from build123d import *

# Parameters (mm, degrees)
BOSS_EXTRUDE1_DEPTH = 3.175
SKETCH2_W           = 11.43
SKETCH2_H           = 100.33
BOSS_EXTRUDE2_DEPTH = 1.5875


with BuildPart() as part:
    # Sketch1 → Boss-Extrude1 (new body)
    with BuildSketch(Plane.XY):
        with BuildLine():
            Line((-50.8, 171.390190343), (-50.8, 171.509809657))
            ThreePointArc((-50.8, 171.509809657), (-52.642354096, 175.957645904), (-57.090190343, 177.8))
            Line((-57.090190343, 177.8), (-190.5, 177.8))
            ThreePointArc((-190.5, 177.8), (-194.990128061, 175.940128061), (-196.85, 171.45))
            Line((-196.85, 171.45), (-196.85, 21.59))
            ThreePointArc((-196.85, 21.59), (-196.106051224, 19.793948776), (-194.31, 19.05))
            Line((-194.31, 19.05), (-193.04, 19.05))
            ThreePointArc((-193.04, 19.05), (-191.243948776, 18.306051224), (-190.5, 16.51))
            Line((-190.5, 16.51), (-190.5, 6.35))
            ThreePointArc((-190.5, 6.35), (-188.640128061, 1.859871939), (-184.15, 0))
            Line((-184.15, 0), (184.15, 0))
            ThreePointArc((184.15, 0), (188.640128061, 1.859871939), (190.5, 6.35))
            Line((190.5, 6.35), (190.5, 16.51))
            ThreePointArc((190.5, 16.51), (191.243948776, 18.306051224), (193.04, 19.05))
            Line((193.04, 19.05), (194.31, 19.05))
            ThreePointArc((194.31, 19.05), (196.106051224, 19.793948776), (196.85, 21.59))
            Line((196.85, 21.59), (196.85, 171.45))
            ThreePointArc((196.85, 171.45), (194.990128061, 175.940128061), (190.5, 177.8))
            Line((190.5, 177.8), (57.090190343, 177.8))
            ThreePointArc((57.090190343, 177.8), (52.642354096, 175.957645904), (50.8, 171.509809657))
            Line((50.8, 171.509809657), (50.8, 171.390190343))
            ThreePointArc((50.8, 171.390190343), (48.957645904, 166.942354096), (44.509809657, 165.1))
            Line((44.509809657, 165.1), (-44.509809657, 165.1))
            ThreePointArc((-44.509809657, 165.1), (-48.957645904, 166.942354096), (-50.8, 171.390190343))
        make_face()
    extrude(amount=BOSS_EXTRUDE1_DEPTH)

    # Sketch2 → Boss-Extrude2 (add)
    with BuildSketch(Plane(origin=(0, 0, 0), x_dir=(-1, 0, 0), z_dir=(0, 0, -1))):
        with Locations((-190.5, 69.215)):
            Rectangle(SKETCH2_W, SKETCH2_H)
        with Locations((190.5, 69.215)):
            Rectangle(SKETCH2_W, SKETCH2_H)
    extrude(amount=BOSS_EXTRUDE2_DEPTH)


solid = part.part
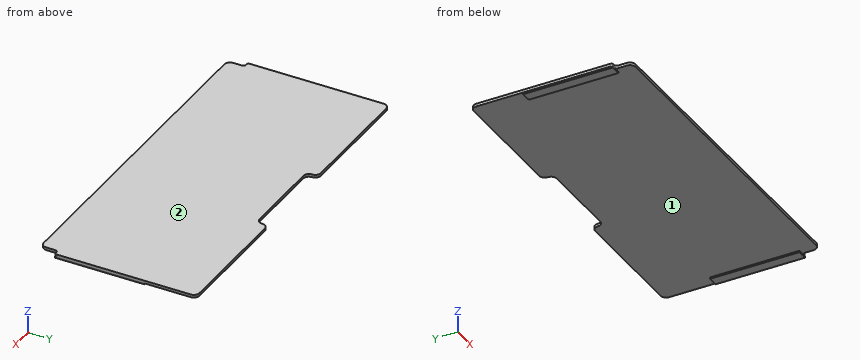
Here's how the part is built. I have some questions about the finished solid (model axes, mm). Face numbers are marked on the shaded views. Coordinates: 2 decimals unless noted, no trailing zeros. Order: outer loops, then holes, each group sorted by start corner. A loop starts at its lowest first (then second) coordinate and runs counter-clockwise, first axis right, second up. Notation, with made-up numbers: (81, 85.5) - (138, 85.5) arc R13 cw to (138, 93.5) - close; hole circle Ø9 at (-4, 69). An arc over 180 degrees is marked (long way). Use CSV: the item, a comma, the result in double quotes. Start each with the question number.
1. Suppose I cut it at A-A on z = -0.75. List the corners of the cut face in (x, y) for me (3 decimals).
2. Suppose I cut it at D-D on x = 11. List the corners of the cut face in (y, z) for me (3 decimals), then the cut area to 3 significant figures.
3. I'm going to push flat-ended pins straight in: pin 1 (0.8 mm diameter, centred on x = 189.5, z = -0.5, fed in from +Y); pin 2 (1.3 mm diameter, centred on y = 45, z = -0.5, fed in from -X); pin 3 (2.5 mm diameter, centred on x = 193, z = 1, fed in from -Y); pin 4 (0.8 mm diameter, centred on y = 57, z = -0.5, fed in from -X) (3 decimals). Where does each tip first touch, or does it pass through?
4. If we mould it in two halves opening along X, with no side actions, what happens to the marked faces 1 and 2? For each: +X half, -X half, draft (parallel to the pull), parting line (faces both ways), or undercut.
5. Suppose I cut it at C-C on x = -108. List the corners of the cut face in (y, z) for me (3 decimals), then the cut area to 3 significant figures.
6. Please list where these lines run through material, in increasing order: line 1 (X direction, y = 32.5, z = -0.65) (3 decimals); line 2 (Z direction, x = -162, y = 141.5) (3 decimals); line 3 (Y direction, x = 6, z = 2.9). Write a range as from..to.
Output:
1,outline,"(-196.215, 19.05) - (-184.785, 19.05) - (-184.785, 119.38) - (-196.215, 119.38) - close; (184.785, 19.05) - (196.215, 19.05) - (196.215, 119.38) - (184.785, 119.38) - close"
2,outline,"(0, 0) - (165.1, 0) - (165.1, 3.175) - (0, 3.175) - close"
2,area,"524 mm2"
3,pin 1,"stops at y = 119.38"
3,pin 2,"stops at x = -196.85"
3,pin 3,"stops at y = 18.7"
3,pin 4,"stops at x = -196.215"
4,face 1,"undercut"
4,face 2,"draft"
5,outline,"(0, 0) - (177.8, 0) - (177.8, 3.175) - (0, 3.175) - close"
5,area,"565 mm2"
6,line 1,"x = -196.215..-184.785, 184.785..196.215"
6,line 2,"z = 0..3.175"
6,line 3,"y = 0..165.1"
